Geometry: see drawing. Coordinates: mm, zero at the bounding-box minimum. Round coordinates to 2 decimals unless told otherwise and drop trailing zeros. Loops run counter-clockwise (first coordinate to the right, second up) from the corner with the lowest first, then second, coordinate; pieces in that order, holes last.
(1) Section B-B, the plane y = 0.55. Count the separate pieces of the cut face and the enclosed holes in it, plus the area to 3 significant figures.
(2) First-contact query: pin 1 Ø1 at (x, z) = (9, 19) entering from -Y. Flat tip, straight axial feed; report the tip coordinate or a pass-through.
(3) Section A-A, the plane x = 5.08. Return the cut outline in (y, z) (1 decimal).
(4) Material intervals for probe 1 along Z at (x, y) = (5.08, 0.4) (1 decimal); probe 2 along X at (y, z) = (0.3, 1) (1 decimal), sorted ascending.
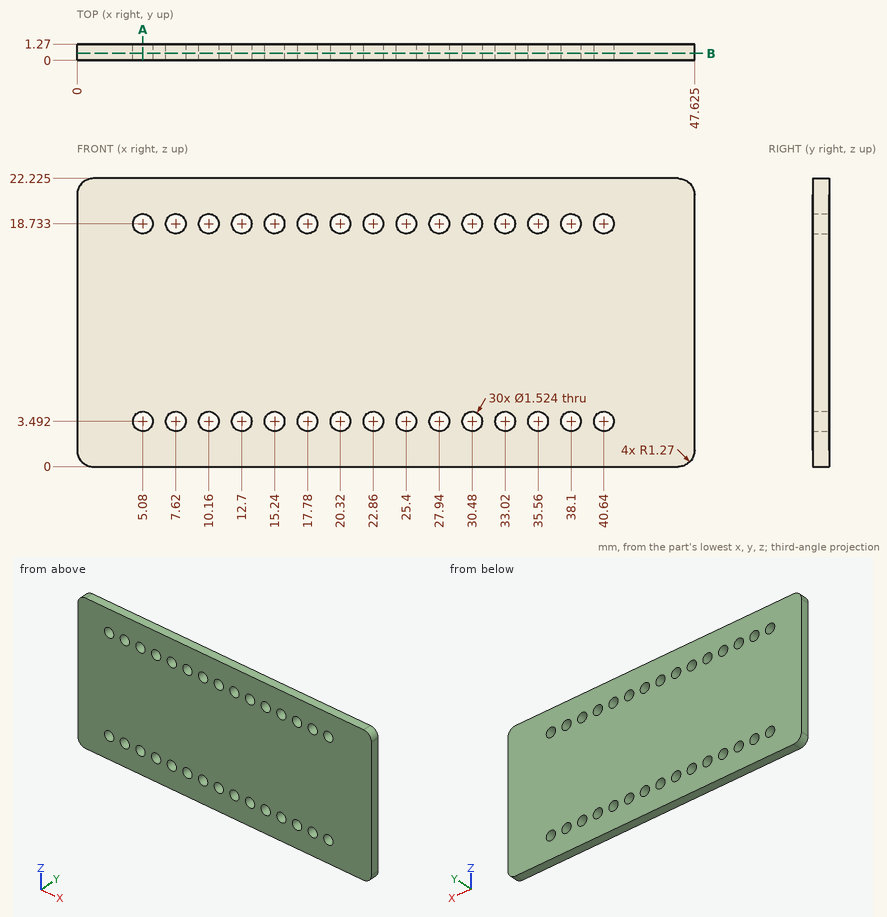
Output values:
1. separate pieces: 1
1. enclosed holes: 30
1. area: 1,000 mm2
2. pin 1: stops at y = 0
3. outline: (0, 0) - (1.3, 0) - (1.3, 2.7) - (0, 2.7) - close; (0, 4.3) - (1.3, 4.3) - (1.3, 18) - (0, 18) - close; (0, 19.5) - (1.3, 19.5) - (1.3, 22.2) - (0, 22.2) - close
4. probe 1: z = 0 to 2.7, 4.3 to 18, 19.5 to 22.2
4. probe 2: x = 0 to 47.6
